CAD build for the part. Positions are in the model's coordinates, mm. A direction names the side the tool comes from. Round coordinates to 2 decimals unless told otherwise and drop trailing zeros. Order: outer loops, then holes, each group sorted by start corner. A loop starts at its lowest first (then second) coordinate and runs counter-clockwise, first axis right, second up. Notation, with made-up numbers: (-6.75, 36) - (45.25, 36) arc R24 cw to (45.25, 50) - close; hole circle Ø6 at (18, 40.5). An arc over 180 degrees is marked (long way). Use one line per item in the form item = value. Start each with the question number.
from build123d import *

# Parameters (mm, degrees)
F3_DEPTH       = 1.5
F4_DEPTH       = 38
F5_START       = 36.5
F5_DEPTH       = 1.5
F7_D           = 4
F7_CSINK_D     = 7
F7_CSINK_ANGLE = 90


with BuildPart() as f3:
    # F2 (on Top) → F3 (new body)
    with BuildSketch(Plane.XY):
        with BuildLine():
            Line((15, 1.5), (15, 0))
            Line((15, 0), (88, 0))
            Line((88, 0), (88, 1.5))
            Line((88, 1.5), (88, 4.5))
            Line((88, 4.5), (98.5, 4.5))
            Line((98.5, 4.5), (98.5, 20))
            Line((98.5, 20), (101.5, 20))
            Line((101.5, 20), (103, 20))
            Line((103, 20), (103, 40))
            ThreePointArc((103, 40), (100.0710678119, 47.0710678119), (93, 50))
            Line((93, 50), (10, 50))
            ThreePointArc((10, 50), (2.9289321881, 47.0710678119), (0, 40))
            Line((0, 40), (0, 20))
            Line((0, 20), (1.5, 20))
            Line((1.5, 20), (4.5, 20))
            Line((4.5, 20), (4.5, 4.5))
            Line((4.5, 4.5), (15, 4.5))
            Line((15, 4.5), (15, 1.5))
        make_face()
        Polygon((1.5, 1.5), (15, 1.5), (15, 4.5), (4.5, 4.5), (4.5, 20), (1.5, 20), align=None)
        Polygon((88, 4.5), (88, 1.5), (101.5, 1.5), (101.5, 20), (98.5, 20), (98.5, 4.5), align=None)
        Polygon((88, 1.5), (88, 0), (103, 0), (103, 20), (101.5, 20), (101.5, 1.5), align=None)
        Polygon((0, 20), (0, 0), (15, 0), (15, 1.5), (1.5, 1.5), (1.5, 20), align=None)
    extrude(amount=F3_DEPTH)

    # F2 (on Top) → F4 (join)
    with BuildSketch(Plane.XY):
        Polygon((0, 20), (0, 0), (15, 0), (15, 1.5), (1.5, 1.5), (1.5, 20), align=None)
        Polygon((88, 1.5), (88, 0), (103, 0), (103, 20), (101.5, 20), (101.5, 1.5), align=None)
    extrude(amount=F4_DEPTH)

    # F2 (on Top) → F5 (join)
    with BuildSketch(Plane.XY.offset(F5_START)):
        Polygon((88, 4.5), (88, 1.5), (101.5, 1.5), (101.5, 20), (98.5, 20), (98.5, 4.5), align=None)
        Polygon((1.5, 1.5), (15, 1.5), (15, 4.5), (4.5, 4.5), (4.5, 20), (1.5, 20), align=None)
    extrude(amount=F5_DEPTH)

    # F7 (through all)
    with Locations(Plane.XY.offset(1.5)):
        with Locations((20, 30), (83, 30)):
            CounterSinkHole(F7_D / 2, F7_CSINK_D / 2, counter_sink_angle=F7_CSINK_ANGLE)


solid = f3.part
(1) Flat gauge pins, fed straight in: P1, Ø8, axis at x = 76.5, y = 19.5, coming from the +Z side; P2, Ø1.3, axis at x = 2.5, z = 29, coming from the +Y side; P3, Ø1.2, axis at x = 92.5, z = 37.5, coming from the +Y side. Where does each tip first touch, or does it go through?
(2) Slice it at B-B (z = 3). Give the cut face in (x, y).
(3) Mould opens along X. For faces 4 (the flat face through (15, 1, 21)), 5 (the flat face through (55, 0, 1)), 6 (the cylindrical face through (3.01, 47.15, 0.74)) say: pulls with the +X half, pulls with the -X half, needs draft (parallel to the pull), parting line crosses it, or undercut.
(4) Which spindle directions (+Z, -Z, +X, -X, +Y, -Y) get a long thin tool onto all of the face, cutting with end or side? Do faces 1 (the flat face through (8, 1.5, 19)), 2 (the flat face through (1, 20, 21)), 3 (the flat face through (88, 1, 21)). Say none if no direction does.
(5) Slice it at C-C (x = 83). Give the cut face in (y, z).
(6) Slice it at A-A (y = 30). Give the cut face in (x, z), and give its area (3 significant figures).
(7) Slice it at D-D (x = 96). Give the cut face in (y, z), and give its area (3 significant figures).
(8) Wall check: line 1 (X direction, y = 7, z = 27); line 2 (Z direction, x = 18.5, y = 39.5). Give the ranges that are in metal, low to high. Write a range as [from, to].
Results list:
q1.P1 = 1.5
q1.P2 = 1.5
q1.P3 = 4.5
q2.outline = (0, 0) - (15, 0) - (15, 1.5) - (1.5, 1.5) - (1.5, 20) - (0, 20) - close; (88, 0) - (103, 0) - (103, 20) - (101.5, 20) - (101.5, 1.5) - (88, 1.5) - close
q3.face_4 = undercut
q3.face_5 = needs draft
q3.face_6 = pulls with the -X half
q4.face_1 = +Y
q4.face_2 = +Z, +X, -X, +Y
q4.face_3 = +Z, +Y, -Y
q5.outline = (0, 0) - (28, 0) - (26.5, 1.5) - (0, 1.5) - close; (32, 0) - (50, 0) - (50, 1.5) - (33.5, 1.5) - close
q6.outline = (0, 0) - (18, 0) - (16.5, 1.5) - (0, 1.5) - close; (22, 0) - (81, 0) - (79.5, 1.5) - (23.5, 1.5) - close; (85, 0) - (103, 0) - (103, 1.5) - (86.5, 1.5) - close
q6.area = 138 mm²
q7.outline = (0, 0) - (49.54, 0) - (49.54, 1.5) - (1.5, 1.5) - (1.5, 36.5) - (4.5, 36.5) - (4.5, 38) - (0, 38) - close
q7.area = 134 mm²
q8.line_1 = [0, 1.5], [101.5, 103]
q8.line_2 = [0, 1.5]
